Study the drawing (mm; zero at the part's minimum x, y, z) and answer. A direction names the side the tool comes from. Round coordinates to 2 decimals unless told otherwise and drop trailing zeros. Write each loop counter-clockwise with the first axis right and the second up, starting at its lowest first coordinate (ties: lowest second). Pieces come first, ordered by that corner, then holes. Notation, with made-up numbers: (59.5, -8.75) -> (79.5, -8.75) arc R18 ccw to (79.5, 26.25) -> close; hole circle Ø4 at (50.5, -7.75). An arc over 180 degrees is marked (long way). Return JSON: item names as keys, results as strings.
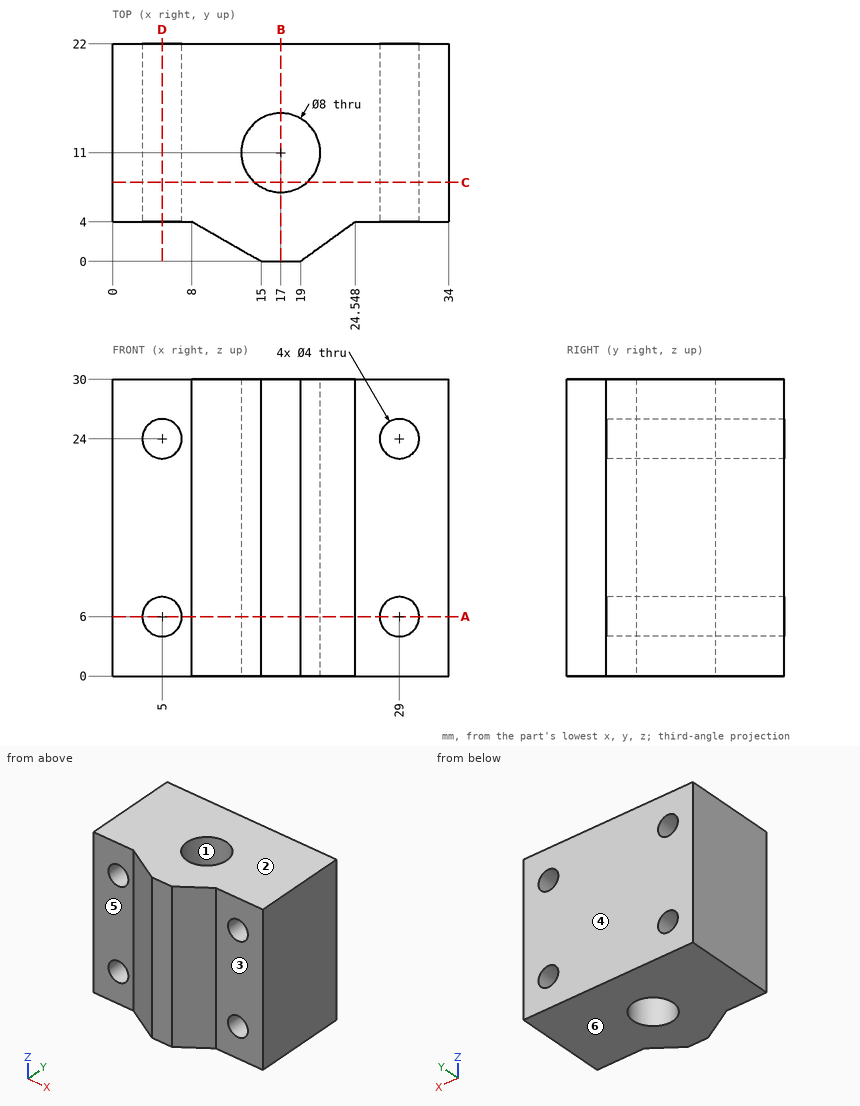
Item 1: Section B-B (x = 17) is taken. Give the vertices of the cut face in (y, z), then the cut area to 3 significant figures.
Worked answers:
{"outline": "(0, 0) -> (7, 0) -> (7, 30) -> (0, 30) -> close; (15, 0) -> (22, 0) -> (22, 30) -> (15, 30) -> close", "area": "420 mm2"}
Item 2: Section C-C (y = 8) is taken. Give the vertices of the cut face in (x, z), then the cut area to 3 significant figures.
Worked answers:
{"outline": "(0, 0) -> (14.35, 0) -> (14.35, 30) -> (0, 30) -> close; (19.65, 0) -> (34, 0) -> (34, 30) -> (19.65, 30) -> close; hole circle Ø4 at (5, 6); hole circle Ø4 at (5, 24); hole circle Ø4 at (29, 6); hole circle Ø4 at (29, 24)", "area": "811 mm2"}
Item 3: Section A-A (z = 6) is taken. Give the vertices of the cut face in (x, y), then the cut area to 3 significant figures.
Worked answers:
{"outline": "(0, 4) -> (3, 4) -> (3, 22) -> (0, 22) -> close; (7, 4) -> (8, 4) -> (15, 0) -> (19, 0) -> (24.55, 4) -> (27, 4) -> (27, 22) -> (7, 22) -> close; (31, 4) -> (34, 4) -> (34, 22) -> (31, 22) -> close; hole circle Ø8 at (17, 11)", "area": "459 mm2"}
Item 4: Straight lines are drawn through the part: L1, parallel to Z at x = 5, y = 18.75; L2, parallel to Z at x = 4, y = 18.5; L3, parallel to X at y = 4.5, z = 5.25. For each, find the intervals that lie inside material, in ascending order. Write a range as [from, to].
Worked answers:
{"L1": "z = [0, 4], [8, 22], [26, 30]", "L2": "z = [0, 4.27], [7.73, 22.27], [25.73, 30]", "L3": "x = [0, 3.15], [6.85, 27.15], [30.85, 34]"}
Item 5: For a pull along Y with two mould halves and no side action, classify the marked faces 1, 2, 3 and 4 as released by +Y, released by -Y, zero draft, split by the parting line, or undercut.
Worked answers:
{"face 1": "undercut", "face 2": "zero draft", "face 3": "released by -Y", "face 4": "released by +Y"}
Item 6: A flat-ended cylindrical pin translates along its axis: pin 1 (5 mm diameter, centred on x = 29, z = 6, fed in from -Y). Find the tip coordinate at first contact, or state that the pin passes through.
Worked answers:
{"pin 1": "stops at y = 4"}
Item 7: Section D-D (x = 5) is taken. Give the vertices of the cut face in (y, z), then the cut area to 3 significant figures.
Worked answers:
{"outline": "(4, 0) -> (22, 0) -> (22, 4) -> (4, 4) -> close; (4, 8) -> (22, 8) -> (22, 22) -> (4, 22) -> close; (4, 26) -> (22, 26) -> (22, 30) -> (4, 30) -> close", "area": "396 mm2"}
Item 8: A tool of negligible diameter and unlimited length cuts with its end or side. For the marked faces 5 and 6, from which of +Z, -Z, +X, -X, +Y, -Y can it reach the whole face along a straight path? Write none if from no direction.
Worked answers:
{"face 5": "+Z, -Z, -X, -Y", "face 6": "-Z, +X, -X, +Y, -Y"}
